```python
from build123d import *

# Parameters (mm, degrees)
BOSS_EXTRUDE1_DEPTH = 50
SHELL1_T            = -3
CUT_EXTRUDE1_DEPTH  = 40
SKETCH3_R           = 2.1
BOSS_EXTRUDE5_DEPTH = 47
SKETCH5_R           = 2
CUT_EXTRUDE2_DEPTH  = 10
BOSS_EXTRUDE6_START = 3
SKETCH6_R           = 6
SKETCH6_R_2         = 2
BOSS_EXTRUDE6_DEPTH = 3
FILLET1_R           = 1
SKETCH7_W           = 32
SKETCH7_H           = 27.7
CUT_EXTRUDE3_DEPTH  = 10
SKETCH8_R           = 6.5
CUT_EXTRUDE4_DEPTH  = 10


with BuildPart() as part:
    # Sketch1 → Boss-Extrude1 (new body)
    with BuildSketch(Plane(origin=(0, 0, 0), x_dir=(1, 0, 0), z_dir=(0, 1, 0))):
        with BuildLine():
            Line((-55, 40), (55, 40))
            ThreePointArc((55, 40), (62.071067812, 37.071067812), (65, 30))
            Line((65, 30), (65, -30))
            ThreePointArc((65, -30), (62.071067812, -37.071067812), (55, -40))
            Line((55, -40), (-55, -40))
            ThreePointArc((-55, -40), (-62.071067812, -37.071067812), (-65, -30))
            Line((-65, -30), (-65, 30))
            ThreePointArc((-65, 30), (-62.071067812, 37.071067812), (-55, 40))
        make_face()
    extrude(amount=BOSS_EXTRUDE1_DEPTH)

    # Shell1
    shell1_openings = [part.faces().sort_by_distance(p)[0] for p in [
        (0, 50, 0),
    ]]
    offset(amount=SHELL1_T, openings=shell1_openings, kind=Kind.INTERSECTION)

    # Sketch2 → Cut-Extrude1 (cut)
    with BuildSketch(Plane.XZ):
        with BuildLine():
            Line((65, -30), (65, 30))
            ThreePointArc((65, 30), (62.071067812, 37.071067812), (55, 40))
            Line((55, 40), (-55, 40))
            ThreePointArc((-55, 40), (-62.071067812, 37.071067812), (-65, 30))
            Line((-65, 30), (-65, -30))
            ThreePointArc((-65, -30), (-62.071067812, -37.071067812), (-55, -40))
            Line((-55, -40), (55, -40))
            ThreePointArc((55, -40), (62.071067812, -37.071067812), (65, -30))
        make_face()
        with BuildLine():
            Line((-63.5, 30), (-63.5, -30))
            ThreePointArc((-63.5, -30), (-61.01040764, -36.01040764), (-55, -38.5))
            Line((-55, -38.5), (55, -38.5))
            ThreePointArc((55, -38.5), (61.01040764, -36.01040764), (63.5, -30))
            Line((63.5, -30), (63.5, 30))
            ThreePointArc((63.5, 30), (61.01040764, 36.01040764), (55, 38.5))
            Line((55, 38.5), (-55, 38.5))
            ThreePointArc((-55, 38.5), (-61.01040764, 36.01040764), (-63.5, 30))
        make_face(mode=Mode.SUBTRACT)
    extrude(amount=-CUT_EXTRUDE1_DEPTH, mode=Mode.SUBTRACT)

    # Sketch5 → Cut-Extrude2 (cut)
    with BuildSketch(Plane(origin=(0, 3, 0), x_dir=(1, 0, 0), z_dir=(0, 1, 0))):
        with Locations(Location((-40, 0, 0), (0, 0, 270))):
            Circle(SKETCH5_R)
        with Locations(Location((40, 0, 0), (0, 0, 270))):
            Circle(SKETCH5_R)
    extrude(amount=-CUT_EXTRUDE2_DEPTH, mode=Mode.SUBTRACT)


with BuildPart() as body_2:
    # Sketch3 → Boss-Extrude5 (new body)
    with BuildSketch(Plane(origin=(0, 3, 0), x_dir=(1, 0, 0), z_dir=(0, 1, 0))):
        with BuildLine():
            Line((62, -30), (62, 30))
            ThreePointArc((62, 30), (59.949747468, 34.949747468), (55, 37))
            Line((55, 37), (-55, 37))
            ThreePointArc((-55, 37), (-59.949747468, 34.949747468), (-62, 30))
            Line((-62, 30), (-62, -30))
            ThreePointArc((-62, -30), (-59.949747468, -34.949747468), (-55, -37))
            Line((-55, -37), (55, -37))
            ThreePointArc((55, -37), (59.949747468, -34.949747468), (62, -30))
        make_face()
        with Locations(Location((-56, 31, 0), (0, 0, 270))):
            Circle(SKETCH3_R, mode=Mode.SUBTRACT)
        with Locations(Location((56, 31, 0), (0, 0, 90))):
            Circle(SKETCH3_R, mode=Mode.SUBTRACT)
        with Locations(Location((56, -31, 0), (0, 0, 270))):
            Circle(SKETCH3_R, mode=Mode.SUBTRACT)
        with Locations(Location((-56, -31, 0), (0, 0, 90))):
            Circle(SKETCH3_R, mode=Mode.SUBTRACT)
        with BuildLine():
            Line((-58.25, 21.75), (-55, 21.75))
            ThreePointArc((-55, 21.75), (-49.343145751, 24.093145751), (-47, 29.75))
            Line((-47, 29.75), (-47, 33.25))
            ThreePointArc((-47, 33.25), (-46.414213562, 34.664213562), (-45, 35.25))
            Line((-45, 35.25), (45, 35.25))
            ThreePointArc((45, 35.25), (46.414213562, 34.664213562), (47, 33.25))
            Line((47, 33.25), (47, 29.75))
            ThreePointArc((47, 29.75), (49.343145751, 24.093145751), (55, 21.75))
            Line((55, 21.75), (58.25, 21.75))
            ThreePointArc((58.25, 21.75), (59.664213562, 21.164213562), (60.25, 19.75))
            Line((60.25, 19.75), (60.25, -19.75))
            ThreePointArc((60.25, -19.75), (59.664213562, -21.164213562), (58.25, -21.75))
            Line((58.25, -21.75), (55, -21.75))
            ThreePointArc((55, -21.75), (49.343145751, -24.093145751), (47, -29.75))
            Line((47, -29.75), (47, -33.25))
            ThreePointArc((47, -33.25), (46.414213562, -34.664213562), (45, -35.25))
            Line((45, -35.25), (-45, -35.25))
            ThreePointArc((-45, -35.25), (-46.414213562, -34.664213562), (-47, -33.25))
            Line((-47, -33.25), (-47, -29.75))
            ThreePointArc((-47, -29.75), (-49.343145751, -24.093145751), (-55, -21.75))
            Line((-55, -21.75), (-58.25, -21.75))
            ThreePointArc((-58.25, -21.75), (-59.664213562, -21.164213562), (-60.25, -19.75))
            Line((-60.25, -19.75), (-60.25, 19.75))
            ThreePointArc((-60.25, 19.75), (-59.664213562, 21.164213562), (-58.25, 21.75))
        make_face(mode=Mode.SUBTRACT)
    extrude(amount=BOSS_EXTRUDE5_DEPTH)


    add(part.part)  # Boss-Extrude6 merges part
    # Sketch6 → Boss-Extrude6 (add)
    # profile 1 of 2: a face of its own
    with BuildSketch(Plane(origin=(0, 3, 0), x_dir=(1, 0, 0), z_dir=(0, 1, 0)).offset(BOSS_EXTRUDE6_START)):
        with Locations(Location((-40, 0, 0), (0, 0, 270))):
            Circle(SKETCH6_R)
        with Locations(Location((-40, 0, 0), (0, 0, 270))):
            Circle(SKETCH6_R_2, mode=Mode.SUBTRACT)
    # profile 2 of 2: a face of its own
    with BuildSketch(Plane(origin=(0, 3, 0), x_dir=(1, 0, 0), z_dir=(0, 1, 0)).offset(BOSS_EXTRUDE6_START)):
        with Locations(Location((40, 0, 0), (0, 0, 90))):
            Circle(SKETCH6_R)
        with Locations(Location((40, 0, 0), (0, 0, 270))):
            Circle(SKETCH6_R_2, mode=Mode.SUBTRACT)
    extrude(amount=-BOSS_EXTRUDE6_DEPTH)

    # Fillet1
    fillet1_edges = [body_2.edges().sort_by_distance(p)[0] for p in [
        (-40, 6, -6),
        (-40, 3, -6),
        (40, 6, 6),
        (40, 3, 6),
    ]]
    fillet(fillet1_edges, radius=FILLET1_R)

    # Sketch7 → Cut-Extrude3 (cut)
    with BuildSketch(Plane.XY.offset(38.5)):
        with Locations((0, 20.830272727)):
            Rectangle(SKETCH7_W, SKETCH7_H)
    extrude(amount=-CUT_EXTRUDE3_DEPTH, mode=Mode.SUBTRACT)

    # Sketch8 → Cut-Extrude4 (cut)
    with BuildSketch(Plane(origin=(0, 0, -38.5), x_dir=(-1, 0, 0), z_dir=(0, 0, -1))):
        with Locations((-32.5, 20)):
            Circle(SKETCH8_R)
        with Locations(Location((32.5, 20, 0), (0, 0, 180))):
            Circle(SKETCH8_R)
    extrude(amount=-CUT_EXTRUDE4_DEPTH, mode=Mode.SUBTRACT)


solid = body_2.part
```
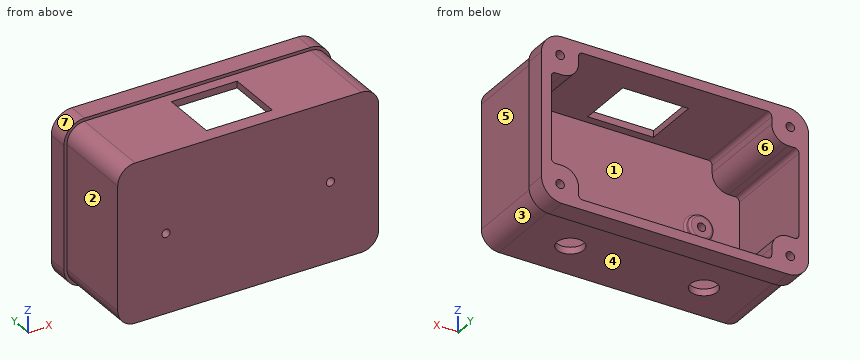
Design review of the part built by this model. Coordinates are the model's own, in mm. Face numbers are marked on the shaded views. A direction names the side the tool comes from. Coordinates: 2 decimals unless noted, no trailing zeros. Order: outer loops, then holes, each group sorted by start corner. A loop starts at its lowest first (then second) coordinate and runs counter-clockwise, first axis right, second up.
1) Take a section at B-B, the plane y = 29.5. State how many separate pieces and enclosed holes the cut face has, and give its area (3 significant figures).
2) Mouldability with a two-part tool opening along Z and no side actions: class the marked faces 5, 6 and 7 as +Z half, -Z half, draft (parallel to the pull), parting line (faces both ways), or undercut.
3) Wall thickness on line 1 along Y through (x, z) = (-3, 36); line 2 along X through (y, z) = (4.5, -17); line 3 along X through (y, z) = (28.5, 31): over which ranges is each line inside the solid? List them lowest first.
4) Take a section at A-A, the plane x = 7.5. Give the boundary of the cut face in (y, z).
5) Clearance check with flat-ended pins moving along their axes: pin 1 (1.6 mm diameter, centred on x = -56.5, y = 17.5, fed in from -Z); pin 2 (1.3 mm diameter, centred on x = -56, z = -31.5, fed in from +Y); pin 3 (1 mm diameter, centred on y = 22, z = -31, fed in from -X); pin 4 (2.5 mm diameter, centred on x = -40, z = 0, fed in from -Y). State where each tip first meets the part, or that it passes through.
6) For the marked faces 1, 2, 3 and 4, list the 3-axis set-ups (+Z, -Z, +X, -X, +Y, -Y) from which the entire face can be reached by the end or side of a thin tool; tool diameter is ignored.
Returned:
1. separate pieces: 1
1. enclosed holes: 4
1. area: 1,730 mm2
2. face 5: draft
2. face 6: undercut
2. face 7: +Z half
3. line 1: y = 0 to 6.98, 34.68 to 50
3. line 2: x = -63.5 to -60.25, 60.25 to 63.5
3. line 3: x = -63.44 to -58.1, -53.9 to -47, 47 to 53.9, 58.1 to 63.44
4. outline: (0, -38.5) - (40, -38.5) - (40, -40) - (50, -40) - (50, -35.25) - (3, -35.25) - (3, 35.25) - (6.98, 35.25) - (6.98, 38.5) - (0, 38.5) - close; (34.68, 35.25) - (50, 35.25) - (50, 40) - (40, 40) - (40, 38.5) - (34.68, 38.5) - close
5. pin 1: stops at z = -38.47
5. pin 2: stops at y = 3
5. pin 3: stops at x = -63.49
5. pin 4: passes through
6. face 1: +Y
6. face 2: +Z, -Z, -X, -Y
6. face 3: -Z, +X, -Y
6. face 4: -Z, +X, -X, -Y
